Here's how the part is built. I have some questions about the finished solid (model axes, mm). Face numbers are marked on the shaded views. Round coordinates to 2 decimals unless told otherwise and drop trailing zeros. Loops run counter-clockwise (first coordinate to the right, second up) from the corner with the lowest first, then second, coordinate; pieces in that order, holes last. Notation, with made-up numbers: M -34.5,79 L 0.5,79 A28 ccw 0.5,116 Z; hole C 52,-27.5 d8. An arc over 180 degrees is marked long. Write each question's results on one line, items separated by ' | '. Start each with the question number.
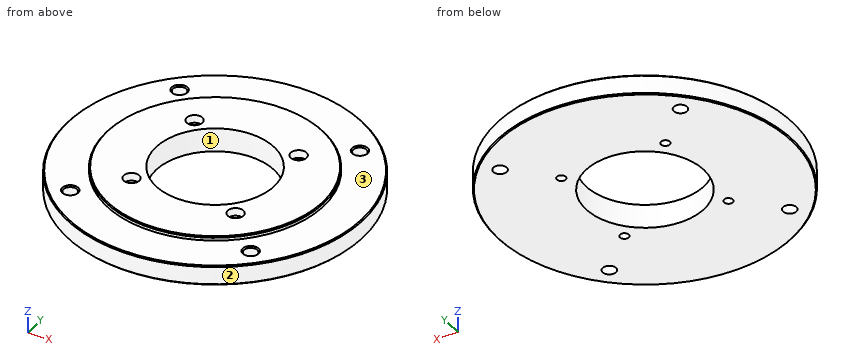
```python
from build123d import *

# Parameters (mm, degrees)
SKETCH1_R                        = 75
BOSS_EXTRUDE1_DEPTH              = 10
SKETCH2_R                        = 55
BOSS_EXTRUDE2_DEPTH              = 2
M8X1_25_TAPPED_HOLE1_D           = 6.8
M8X1_25_TAPPED_HOLE1_CSINK_D     = 8.05
M8X1_25_TAPPED_HOLE1_CSINK_ANGLE = 90
CHAMFER1_SIZE                    = 0.5
SKETCH5_R                        = 30
CUT_EXTRUDE1_DEPTH               = 107.742681248
CBORE_FOR_M4_SHCS1_D             = 4.5
CBORE_FOR_M4_SHCS1_CBORE_D       = 8
CBORE_FOR_M4_SHCS1_CBORE_DEPTH   = 4


with BuildPart() as part:
    # Sketch1 → Boss-Extrude1 (new body)
    with BuildSketch(Plane.XY):
        Circle(SKETCH1_R)
    extrude(amount=BOSS_EXTRUDE1_DEPTH)

    # Sketch2 → Boss-Extrude2 (add)
    with BuildSketch(Plane.XY.offset(10)):
        Circle(SKETCH2_R)
    extrude(amount=BOSS_EXTRUDE2_DEPTH)

    # M8x1.25 Tapped Hole1 (through all)
    with Locations(Plane(origin=(-45.961940777, 45.961940777, 10), x_dir=(1, 0, 0), z_dir=(0, 0, 1))):
        with Locations((0, 0), (91.923881554, 0), (0, -91.923881554), (91.923881554, -91.923881554)):
            CounterSinkHole(M8X1_25_TAPPED_HOLE1_D / 2, M8X1_25_TAPPED_HOLE1_CSINK_D / 2, counter_sink_angle=M8X1_25_TAPPED_HOLE1_CSINK_ANGLE)

    # Chamfer1
    chamfer1_edges = [part.edges().sort_by_distance(p)[0] for p in [
        (-75, 0, 0),
        (-75, 0, 10),
        (-55, 0, 12),
    ]]
    chamfer(chamfer1_edges, length=CHAMFER1_SIZE)

    # Sketch5 → Cut-Extrude1 (cut, through all)
    with BuildSketch(Plane(origin=(0, 0, 0), x_dir=(-1, 0, 0), z_dir=(0, 0, -1))):
        Circle(SKETCH5_R)
    extrude(amount=-CUT_EXTRUDE1_DEPTH, mode=Mode.SUBTRACT)

    # CBORE for M4 SHCS1 (through all)
    with Locations(Plane(origin=(-26.516504294, 26.516504294, 12), x_dir=(1, 0, 0), z_dir=(0, 0, 1))):
        with Locations((0, 0), (53.033008588, 0), (0, -53.033008588), (53.033008588, -53.033008588)):
            CounterBoreHole(CBORE_FOR_M4_SHCS1_D / 2, CBORE_FOR_M4_SHCS1_CBORE_D / 2, CBORE_FOR_M4_SHCS1_CBORE_DEPTH)


solid = part.part
```
1. I need wall thicknesses on line 1 along X through (y, z) = (-24.5, 9.25); line 2 along X through (y, z) = (43, 4.5); line 3 along X through (y, z) = (-27.5, 8.25). Which ranges of each line are inside material? Lowest first, please.
2. I want a section at A-A on y = 0. List the corners of the cut face in (x, z) for me.
3. I want a section at C-C on z = 6.25. Count the separate pieces of the cut face and the enclosed holes in it, plus the area to 3 significant figures.
4. For pin 1 (2.5 mm diameter, centred on x = -25, y = -27, fed in from +Z); pin 2 (3 mm diameter, centred on x = 26.5, z = 10, fed in from -Y); pin 3 (5 mm diameter, centred on x = 5, z = 7.5, fed in from -Y), each with a flat end and sliding along its axis, tell me the tip position at first contact or that it passes through.
5. If we mould it in two halves opening along Y, with no side actions, what happens to the marked faces 1, 2 and 3? For each: released by +Y, released by -Y, zero draft, split by the parting line, or undercut.
Outcome:
1) line 1: -70.89 to -29.97, -23.06 to -17.31, 17.31 to 23.06, 29.97 to 70.89 | line 2: -61.45 to -47.63, -44.29 to 44.29, 47.63 to 61.45 | line 3: -69.78 to -30.39, -22.64 to -11.99, 11.99 to 22.64, 30.39 to 69.78
2) outline: M -75,0.5 L -74.5,0 L -30,0 L -30,12 L -54.5,12 L -55,11.5 L -55,10 L -74.5,10 L -75,9.5 Z; M 30,0 L 74.5,0 L 75,0.5 L 75,9.5 L 74.5,10 L 55,10 L 55,11.5 L 54.5,12 L 30,12 Z
3) separate pieces: 1 | enclosed holes: 9 | area: 14,600 mm2
4) pin 1: z = 8 | pin 2: y = -70.68 | pin 3: y = -74.96
5) face 1: undercut | face 2: split by the parting line | face 3: zero draft
